Here's how the part is built. I have some questions about the finished solid (model axes, mm). A direction names the side the tool comes from. Round coordinates to 2 decimals unless told otherwise and drop trailing zeros. Write each loop counter-clockwise with the first axis right and the second up, starting at its lowest first coordinate (ties: lowest second). Pieces come first, ordered by that corner, then holes. Notation, with made-up numbers: (78.25, -5) -> (98.25, -5) arc R12 cw to (98.25, 13) -> close; hole circle Ø10 at (73, 61.25). An arc over 180 degrees is marked (long way). Answer as CSV lines item,"result".
Autodesk Inventor part; units mm, degrees
ref_plane "YZ Plane" through (0, 0, 0) normal (1, 0, 0) x (0, 1, 0)
ref_plane "XZ Plane" through (0, 0, 0) normal (0, 1, 0) x (-1, 0, 0)
ref_plane "XY Plane" through (0, 0, 0) normal (0, 0, 1) x (1, 0, 0)
sketch "Sketch1" plane through (0, 0, 0) normal (1, 0, 0) x (0, 1, 0)
  line L0 (13.5, 9.5) -> (8, 15)
  line L1 (8, 15) -> (0, 15)
  line L2 (0, 15) -> (0, -15)
  line L3 (8, -15) -> (13.5, -9.5)
  line L4 (13.5, -9.5) -> (13.5, 9.5)
  line L5 (0, -15) -> (8, -15)
  point P0 (0, 0)
  dimension "d21" = 30
  dimension "d22" = 8
  dimension "d23" = 13.5
extrude "Extrusion2" add sketch "Sketch1" along normal blind 10
sketch "Sketch2" plane through (10, 0, 0) normal (1, 0, 0) x (0, 0, -1)
  line L0 (4.5621, 0) -> (7.4708, 0)
  arc A0 (4.5621, 0) -> (-4.5621, 0) centre (0, 3.5) ccw
  arc A1 (7.4708, 0) -> (-7.4708, 0) centre (0, 3.5) ccw
  line L1 (-7.4708, 0) -> (-4.5621, 0)
  line L2 (-15, 0) -> (15, 0)
  point P0 (0, 0)
  dimension "d18" = 5.75
  dimension "d19" = 3.5
  dimension "d20" = 8.25
extrude "Extrusion1" cut sketch "Sketch2" against normal blind 4.3 contours A0 L1 A1 L0
hole "Hole2" at (0, 4, -12) direction (1, 0, 0) diameter 4.5 depth 10
sketch "Sketch3" plane through (0, 0, 0) normal (1, 0, 0) x (0, 1, 0)
  point P0 (4, -12)
hole "Hole1" at (0, 4, 12) direction (1, 0, 0) diameter 4.5 depth 10
sketch "Sketch4" plane through (0, 0, 0) normal (1, 0, 0) x (0, 1, 0)
  point P0 (4, 12)
properties part number "Spreader Holder" material "ASA Plastic"
Item 1: Will this pin go through, and if not, where does the flat tip stop? pin 1 (2 mm diameter, centred on x = 3, y = 9.5, fed in from -Z).
Results found:
pin 1,"stops at z = -14.5"
Item 2: Suppose I cut it at A-A, the plane z = 12. List the corners of the cut face in (x, y) for me.
Results found:
outline,"(0, 0) -> (10, 0) -> (10, 1.75) -> (0, 1.75) -> close; (0, 6.25) -> (10, 6.25) -> (10, 11) -> (0, 11) -> close"
Item 3: Suppose I cut it at B-B, the plane x = 6. List the corners of the cut face in (y, z) for me.
Results found:
outline,"(0, -15) -> (8, -15) -> (13.5, -9.5) -> (13.5, 9.5) -> (8, 15) -> (0, 15) -> (0, 7.47) arc R8.25 cw (long way) to (0, -7.47) -> close; (0, -4.56) arc R5.75 ccw (long way) to (0, 4.56) -> close; hole circle Ø4.5 at (4, -12); hole circle Ø4.5 at (4, 12)"
Item 4: If we mould it in two halves opening along Z, with no side actions, what happens to faces 1 (the cylindrical face through (7.88, 9.247, -0.179)), 2 (the flat face through (5, 11, 12)), 3 (the flat face through (0, 7, 0))? For each: pulls with the +Z half, pulls with the -Z half, needs draft (parallel to the pull), parting line crosses it, or undercut.
Results found:
face 1,"undercut"
face 2,"pulls with the +Z half"
face 3,"needs draft"
Item 5: I need wall thicknesses on L1, parallel to Z at x = 5, y = 4; L2, parallel to Z at x = 8.25, y = 4; L3, parallel to Z at x = 4, y = 2. Which ranges of each line are inside material? Lowest first, please.
Results found:
L1,"z = -15 to -14.25, -9.75 to 9.75, 14.25 to 15"
L2,"z = -15 to -14.25, -9.75 to -8.23, -5.73 to 5.73, 8.23 to 9.75, 14.25 to 15"
L3,"z = -15 to -13.03, -10.97 to 10.97, 13.03 to 15"
Item 6: Suppose I cut it at C-C, the plane y = 3.5. List the corners of the cut face in (x, z) for me.
Results found:
outline,"(0, -15) -> (10, -15) -> (10, -14.19) -> (0, -14.19) -> close; (0, -9.81) -> (10, -9.81) -> (10, -8.25) -> (5.7, -8.25) -> (5.7, -5.75) -> (10, -5.75) -> (10, 5.75) -> (5.7, 5.75) -> (5.7, 8.25) -> (10, 8.25) -> (10, 9.81) -> (0, 9.81) -> close; (0, 14.19) -> (10, 14.19) -> (10, 15) -> (0, 15) -> close"
Item 7: For faces 4 (the flat face through (10, 13, 0)), 5 (the flat face through (5.7, 10, 0)), which set-ups out of +Z, -Z, +X, -X, +Y, -Y let a thin tool reach every point of the face, with its end or its side?
Results found:
face 4,"+Z, -Z, +X, +Y, -Y"
face 5,"+X"
Item 8: Suppose I cut it at D-D, the plane z = 0. List the corners of the cut face in (x, y) for me, then the cut area to 3 significant figures.
Results found:
outline,"(0, 0) -> (10, 0) -> (10, 9.25) -> (5.7, 9.25) -> (5.7, 11.75) -> (10, 11.75) -> (10, 13.5) -> (0, 13.5) -> close"
area,"124 mm²"
